Geometry: final body of the model. Coordinates: model frame, mm. Face numbers are marked on the shaded views. A direction names the side the tool comes from. Give positions to 0.01 mm unless a question says otherwise; leave off trailing zeros. Write each loop counter-clockwise with the first axis right and the second up, starting at its lowest first coordinate (ties: lowest second). Pieces come first, ordered by that corner, then holes. Notation, with made-up numbers: M -33.75,25 L 16.25,25 A9 cw 16.25,29 Z; hole C 27.5,-4 d10. An arc over 180 degrees is marked long. Answer as a JSON object with one key per item and string values.
from build123d import *

# Parameters (mm, degrees)
F0_W        = 40
F0_H        = 30
F1_DEPTH    = 6.25
F2_R        = 5
F3_W        = 5
F3_H        = 25
F4_DEPTH    = 20
F5_T1_DEPTH = 5
F5_T3_DEPTH = 5
F5_T5_DEPTH = 30
F5_T7_DEPTH = 30
F7_R        = 5
F8_DEPTH    = 5
F6_R        = 3.275
F9_DEPTH    = 25
F10_W       = 2.5
F10_H       = 30
F11_DEPTH   = 2


# Not quite as in the source:
# - a fillet or chamfer that OpenCascade refuses, or shapes differently, is made with other operations: its cross-section is extruded or revolved along the edge and cut away or added


with BuildPart() as f1:
    # F0 (on Top) → F1 (new body)
    with BuildSketch(Plane.XY):
        with Locations((1.2747282162, -9.7165126197)):
            Rectangle(F0_W, F0_H)
    extrude(amount=F1_DEPTH)

    # F2
    f2_edges = [f1.edges().sort_by_distance(p)[0] for p in [
        (-18.725272, -24.716513, 3.125),
        (21.274728, -24.716513, 3.125),
        (21.274728, 5.283487, 3.125),
        (-18.725272, 5.283487, 3.125),
    ]]
    fillet(f2_edges, radius=F2_R)

    # F3 (on face) → F4 (join)
    with BuildSketch(Plane.XY.offset(6.25)):
        with Locations((1.2747282162, -9.7165126197)):
            Rectangle(F3_W, F3_H)
    extrude(amount=F4_DEPTH)

    # F5: fillet of radius 5 on 4 edges, made by hand

    # F5_s2 → F5_t1 (join)
    with BuildSketch(Plane.YZ.offset(-1.2252717838)):
        with BuildLine():
            ThreePointArc((5.2834873803, 6.25), (3.4533603614, 8.0801270189), (2.7834873803, 10.5801270189))
            Line((2.7834873803, 10.5801270189), (2.7834873803, 6.25))
            Line((2.7834873803, 6.25), (5.2834873803, 6.25))
        make_face()
    extrude(amount=F5_T1_DEPTH)

    # F5_s4 → F5_t3 (join)
    with BuildSketch(Plane.YZ.offset(-1.2252717838)):
        with BuildLine():
            ThreePointArc((-24.7165126197, 6.25), (-22.8863856008, 8.0801270189), (-22.2165126197, 10.5801270189))
            Line((-22.2165126197, 10.5801270189), (-22.2165126197, 6.25))
            Line((-22.2165126197, 6.25), (-24.7165126197, 6.25))
        make_face()
    extrude(amount=F5_T3_DEPTH)

    # F5_s6 → F5_t5 (cut)
    with BuildSketch(Plane.YZ.offset(-13.7252717838)):
        with BuildLine():
            ThreePointArc((2.7834873803, 21.25), (1.3190212862, 24.7855339059), (-2.2165126197, 26.25))
            Line((-2.2165126197, 26.25), (2.7834873803, 26.25))
            Line((2.7834873803, 26.25), (2.7834873803, 21.25))
        make_face()
    extrude(amount=F5_T5_DEPTH, mode=Mode.SUBTRACT)

    # F5_s8 → F5_t7 (cut)
    with BuildSketch(Plane.YZ.offset(-13.7252717838)):
        with BuildLine():
            ThreePointArc((-22.2165126197, 21.25), (-20.7520465256, 24.7855339059), (-17.2165126197, 26.25))
            Line((-17.2165126197, 26.25), (-22.2165126197, 26.25))
            Line((-22.2165126197, 26.25), (-22.2165126197, 21.25))
        make_face()
    extrude(amount=F5_T7_DEPTH, mode=Mode.SUBTRACT)

    # F7 (on face) → F8 (cut)
    with BuildSketch(Plane.YZ.offset(3.7747282162)):
        with Locations((-9.7165126197, 15.9150635095)):
            Circle(F7_R)
    extrude(amount=-F8_DEPTH, mode=Mode.SUBTRACT)

    # F6 (on face) → F9 (cut)
    with BuildSketch(Plane.XY.offset(6.25)):
        with Locations((-13.7252717838, -1.2665126197)):
            Circle(F6_R)
        with Locations((-13.7252717838, -18.1665126197)):
            Circle(F6_R)
    extrude(amount=-F9_DEPTH, mode=Mode.SUBTRACT)

    # F10 (on face) → F11 (cut)
    with BuildSketch(Plane(origin=(0, 0, 0), x_dir=(1, 0, 0), z_dir=(0, 0, -1))):
        with Locations((11.3062032312, 9.7165126197)):
            Rectangle(F10_W, F10_H)
    extrude(amount=-F11_DEPTH, mode=Mode.SUBTRACT)


solid = f1.part
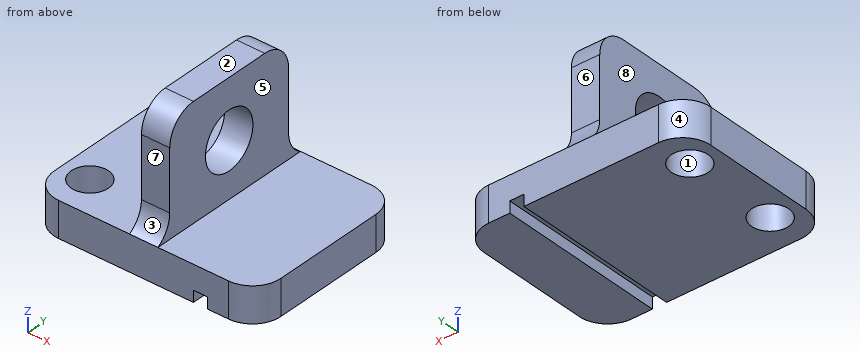
1) Cut plane A-A on y = -9. Return loops of the section in (x, z), and give its area (3 significant figures).
Geometry check:
{"outline": "M -18.73,0 L 10.06,0 L 10.06,2 L 12.56,2 L 12.56,0 L 21.27,0 L 21.27,6.25 L 3.77,6.25 L 3.77,10.97 L -1.23,10.97 L -1.23,6.25 L -18.73,6.25 Z; M -1.23,20.86 L 3.77,20.86 L 3.77,26.25 L -1.23,26.25 Z", "area": "296 mm2"}
2) Cut plane C-C on z = 14.5. Return loops of the section in (x, y).
Geometry check:
{"outline": "M -1.23,-22.22 L 3.77,-22.22 L 3.77,-14.51 L -1.23,-14.51 Z; M -1.23,-4.92 L 3.77,-4.92 L 3.77,2.78 L -1.23,2.78 Z"}
3) Cut plane D-D on x = 5.5. Return loops of the section in (y, z).
Geometry check:
{"outline": "M -24.72,0 L 5.28,0 L 5.28,6.25 L -24.72,6.25 Z"}
4) Pull-direction query (Y, two-part tool) for the marked faces 1, 2 and 3; classes: pulls with the +Y half, pulls with the -Y half, needs draft (parallel to the pull), parting line crosses it, or undercut.
Geometry check:
{"face 1": "undercut", "face 2": "needs draft", "face 3": "pulls with the -Y half"}
5) Line query: line 1 (X direction, y = -7, z = 1.5); line 2 (Z direction, x = 8, y = -12); line 3 (Z direction, x = 11, y = -2.5). Output: solid intervals per line, ascending. Write a range as from..to.
Geometry check:
{"line 1": "x = -18.73..10.06, 12.56..21.27", "line 2": "z = 0..6.25", "line 3": "z = 2..6.25"}
6) Cut plane B-B on x = -15. Return loops of the section in (y, z), and give its area (3 significant figures).
Geometry check:
{"outline": "M -24.55,0 L -21.18,0 L -21.18,6.25 L -24.55,6.25 Z; M -15.15,0 L -4.28,0 L -4.28,6.25 L -15.15,6.25 Z; M 1.75,0 L 5.12,0 L 5.12,6.25 L 1.75,6.25 Z", "area": "110 mm2"}
7) Contact query for flat-ended pins moving along their axis: P1, Ø14, axis at x = 12, y = -2.5, coming from the +Z side; P2, Ø4, axis at x = 0.5, z = 15, coming from the +Y side; P3, Ø3, axis at x = 5.5, z = 10.5, coming from the -Y side; P4, Ø0.8, axis at x = 11, y = -12.5, coming from the -Z side. Output: stop coordinate, or through.
Geometry check:
{"P1": "stops at z = 6.25", "P2": "stops at y = 2.78", "P3": "passes through", "P4": "stops at z = 2"}
8) Set-up query: the marked faces 4, 5, 6, 7 and 8. Return all of +Z, -Z, +X, -X, +Y, -Y with unobstructed straight access to the full face (end or side cutting, diameter ignored); none if empty.
Geometry check:
{"face 4": "+Z, -Z, -X, +Y", "face 5": "+Z, +X, +Y, -Y", "face 6": "+Z, +X, -X, +Y", "face 7": "+Z, +X, -X, -Y", "face 8": "+Z, -X, +Y, -Y"}
